Source: CAD feature listing. Evaluate the final solid. Frame: model axes, mm. Give positions to 0.01 mm unless a question says otherwise; leave off trailing zeros. Order: outer loops, then holes, each group sorted by start corner. A loop starts at its lowest first (then second) coordinate and runs counter-clockwise, first axis right, second up. Notation, with made-up numbers: (-35.5, -37) - (-13.5, -37) arc R11 ccw to (-13.5, -30) - close; hole circle Ø2 at (57.25, -30.75). An arc over 180 degrees is marked (long way). Use CSV: the item, a comma, the result in double quotes.
Autodesk Inventor part; units mm, degrees
ref_plane "YZ Plane" through (0, 0, 0) normal (1, 0, 0) x (0, 1, 0)
ref_plane "XZ Plane" through (0, 0, 0) normal (0, 1, 0) x (-1, 0, 0)
ref_plane "XY Plane" through (0, 0, 0) normal (0, 0, 1) x (1, 0, 0)
sketch "Sketch1" plane through (0, 0, 0) normal (1, 0, 0) x (0, 1, 0)
  line L0 (20, 0) -> (-20, 0) construction
  line L1 (0, 20) -> (0, -20) construction
  line L2 (0, 0) -> (0, -10)
  line L3 (0, 0) -> (14, 0)
  line L4 (0, -10) -> (14, -1.9171)
  line L5 (14, 0) -> (14, -1.9171)
  dimension "d1" = 40
  dimension "d2" = 40
  dimension "d5" = 90
  dimension "d6" = 60
  dimension "d7" = 30
  dimension "d8" = 10
  dimension "squared_surface" = 14
extrude "Extrusion1" add sketch "Sketch1" along normal blind 14
chamfer "Chamfer1" distance 1.75 angle 45 1 edges at (0, 14, -0.9585)
chamfer "Chamfer2" distance 1.75 angle 45 1 edges at (14, 14, -0.9585)
equation "\"d10\" = squared_surface"
properties part number "anamorphic_prism_caf2" material "Glass"
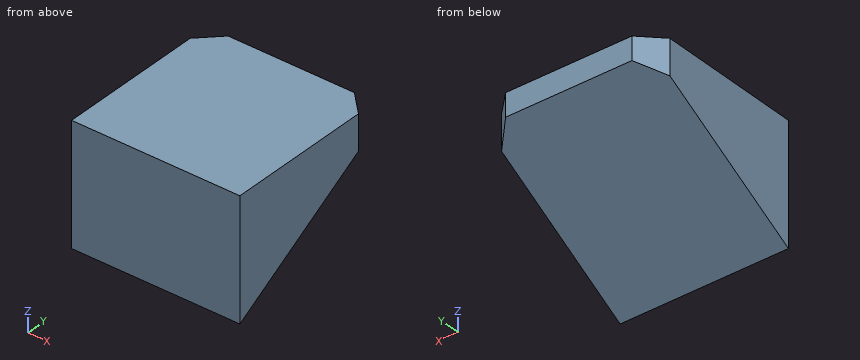
Item 1: Section A-A on z = -1.25. Return the cut outline in (x, y).
Filled in:
outline,"(0, 0) - (14, 0) - (14, 12.25) - (12.25, 14) - (1.75, 14) - (0, 12.25) - close"
Item 2: Material intervals for line 1 (Z direction, x = 8, y = 10.5); line 2 (Y direction, x = 7, z = -5.75); line 3 (Y direction, x = 3.5, z = -5.5), sorted ascending. Write a range as from..to.
Filled in:
line 1,"z = -3.94..0"
line 2,"y = 0..7.36"
line 3,"y = 0..7.79"
Item 3: Section C-C on x = 11.25. Return the cut outline in (y, z), then the cut area to 3 significant figures.
Filled in:
outline,"(0, -10) - (14, -1.92) - (14, 0) - (0, 0) - close"
area,"83.4 mm2"
Item 4: First-contact query: pin 1 (1 mm diameter, centred on x = 6.5, y = 11.5, fed in from -Z); pin 2 (1.5 mm diameter, centred on x = 7.5, z = -4, fed in from +Y); pin 3 (4 mm diameter, centred on y = 8.5, z = -8, fed in from -X); pin 4 (4 mm diameter, centred on x = 7.5, y = 10, fed in from -Z). Flat tips, straight axial feed; report the tip coordinate or a pass-through.
Filled in:
pin 1,"stops at z = -3.65"
pin 2,"stops at y = 11.69"
pin 3,"passes through"
pin 4,"stops at z = -5.38"
Item 5: Section B-B on y = 4.25. Return the cut outline in (x, z), then the cut area to 3 significant figures.
Filled in:
outline,"(0, -7.55) - (14, -7.55) - (14, 0) - (0, 0) - close"
area,"106 mm2"
